Autodesk Inventor part; units mm, degrees
ref_plane "YZ Plane" through (0, 0, 0) normal (1, 0, 0) x (0, 1, 0)
ref_plane "XZ Plane" through (0, 0, 0) normal (0, 1, 0) x (-1, 0, 0)
ref_plane "XY Plane" through (0, 0, 0) normal (0, 0, 1) x (1, 0, 0)
sketch "Boceto1" plane through (0, 0, 0) normal (0, 1, 0) x (-1, 0, 0)
  line L0 (-10, 30) -> (10, 30)
  line L1 (10, 30) -> (10, -30)
  line L2 (10, -30) -> (-10, -30)
  line L3 (-10, -30) -> (-10, 30)
  line L4 (-10, 30) -> (10, -30) construction
  line L5 (10, 30) -> (-10, -30) construction
  circle A0 centre (0, 0) radius 3
  dimension "d0" = 6
  dimension "d1" = 60
  dimension "d2" = 20
extrude "Extrusión1" add sketch "Boceto1" along normal blind 10
sketch "Boceto2" plane through (0, 0, 0) normal (0, -1, 0) x (1, 0, 0)
  circle A0 centre (0, 13) radius 2.7
  circle A1 centre (0, -13) radius 2.7
  point P0 (0, 0)
  dimension "d5" = 5.4
  dimension "d6" = 13
  dimension "d7" = 13
extrude "Extrusión2" cut sketch "Boceto2" against normal through all
sketch "Boceto3" plane through (0, 0, 0) normal (0, -1, 0) x (1, 0, 0)
  line L0 (-6.5, 25.5) -> (6.5, 25.5)
  line L1 (6.5, 25.5) -> (6.5, -25.5)
  line L2 (6.5, -25.5) -> (-6.5, -25.5)
  line L3 (-6.5, -25.5) -> (-6.5, 25.5)
  circle A0 centre (0, 0) radius 3
  line L4 (-6.5, 25.5) -> (6.5, -25.5) construction
  line L5 (6.5, 25.5) -> (-6.5, -25.5) construction
  circle A1 centre (0, -13) radius 2.7
  circle A2 centre (0, 13) radius 2.7
  line L6 (10, -30) -> (-10, -30)
  line L7 (10, 30) -> (10, -30)
  line L8 (-10, 30) -> (10, 30)
  line L9 (-10, -30) -> (-10, 30)
  circle A3 centre (0, 0) radius 3
  dimension "d10" = 51
  dimension "d11" = 13
extrude "Extrusión3" add sketch "Boceto3" along normal blind 10 contours L6 L9 L8 L7
sketch "Boceto4" plane through (0, 10, 0) normal (0, 1, 0) x (1, 0, 0)
  circle A0 centre (0, 0) radius 6
  dimension "d14" = 12
extrude "Extrusión4" cut sketch "Boceto4" against normal blind 6
properties part number "LoadCellUpperPiece"
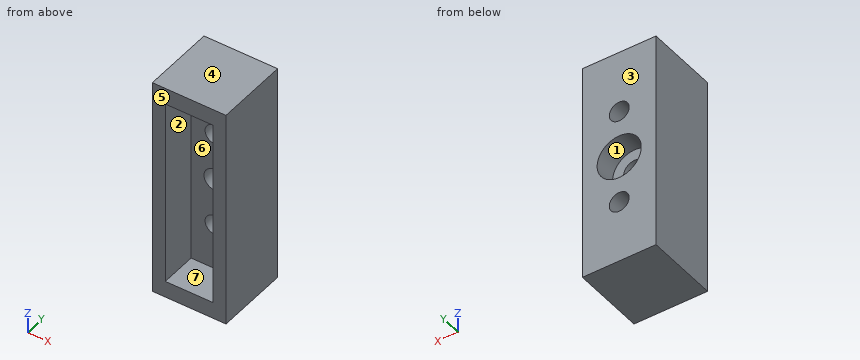
Part model, mm, in its own coordinate system. Face numbers are marked on the shaded views. A direction names the side the tool comes from. Coordinates: 2 decimals unless noted, no trailing zeros. Write each loop counter-clockwise with the first axis right and the second up, starting at its lowest first coordinate (ties: lowest second). Pieces come first, ordered by that corner, then holes. Notation, with made-up numbers: M 0.25,-5 L 31.25,-5 A31 cw 31.25,27 Z; hole C -38,12.25 d7. An arc over 180 degrees is marked long. Return JSON: item names as keys, results as strings.
1. Pull direction Z, two halves, no side cores. Call the marked faces 4, 5, 6 and 7: pulls with the +Z half, pulls with the -Z half, needs draft (parallel to the pull), parting line crosses it, or undercut.
Determined:
{"face 4": "pulls with the +Z half", "face 5": "needs draft", "face 6": "undercut", "face 7": "undercut"}
2. Saw through at D-D, the plane y = 6.5. Write the cut outline in (x, z), then the cut area to 3 significant figures.
Determined:
{"outline": "M -10,-30 L 10,-30 L 10,30 L -10,30 Z; hole C 0,0 d12; hole C 0,-13 d5.4; hole C 0,13 d5.4", "area": "1,040 mm²"}
3. Saw through at B-B, the plane z = 13. Write the cut outline in (x, y), then the cut area to 3 significant figures.
Determined:
{"outline": "M -10,-10 L -6.5,-10 L -6.5,0 L -2.7,0 L -2.7,10 L -10,10 Z; M 2.7,0 L 6.5,0 L 6.5,-10 L 10,-10 L 10,10 L 2.7,10 Z", "area": "216 mm²"}
4. Flat gauge pins, fed straight in: pin 1 Ø9.5 at (x, z) = (-2, 2) entering from +Y; pin 2 Ø5.5 at (x, z) = (0, 0) entering from -Y; pin 3 Ø11 at (x, z) = (0, 0) entering from -Y. Where does each tip first touch, or does it go through?
Determined:
{"pin 1": "y = 10", "pin 2": "through", "pin 3": "y = 0"}
5. Probe L1, parallel to Z at x = 0, y = 8.7; L2, parallel to X at y = 5.2, z = 0; L3, parallel to X at y = -2, z = -22. List the from-to ranges inside material, lowest first.
Determined:
{"L1": "-30 to -15.7, -10.3 to -6, 6 to 10.3, 15.7 to 30", "L2": "-10 to -6, 6 to 10", "L3": "-10 to -6.5, 6.5 to 10"}
6. 3-axis set-ups, long thin cutter, end or side, ignore diameter. For the marked faces 1, 2 and 3: which of +Z, -Z, +X, -X, +Y, -Y reach the whole face in a straight line?
Determined:
{"face 1": "+Y", "face 2": "-Y", "face 3": "+Z, -Z, +X, -X, +Y"}
7. Saw through at C-C, the plane y = -5.5. Write the cut outline in (x, z), then the cut area to 3 significant figures.
Determined:
{"outline": "M -10,-30 L 10,-30 L 10,30 L -10,30 Z; hole M -6.5,-25.5 L 6.5,-25.5 L 6.5,25.5 L -6.5,25.5 Z", "area": "537 mm²"}
8. Saw through at A-A, the plane x = 0. Write the cut outline in (y, z).
Determined:
{"outline": "M -10,-30 L 10,-30 L 10,-15.7 L 0,-15.7 L 0,-25.5 L -10,-25.5 Z; M -10,25.5 L 0,25.5 L 0,15.7 L 10,15.7 L 10,30 L -10,30 Z; M 0,-10.3 L 10,-10.3 L 10,-6 L 4,-6 L 4,-3 L 0,-3 Z; M 0,3 L 4,3 L 4,6 L 10,6 L 10,10.3 L 0,10.3 Z"}
